Verification items for the finished model (mm, model axes). Face numbers are marked on the shaded views. A direction names the side the tool comes from. Round coordinates to 2 decimals unless told otherwise and drop trailing zeros. Write each loop counter-clockwise with the first axis right and the second up, starting at its lowest first coordinate (ties: lowest second). Pieces come first, ordered by that corner, then holes. Notation, with made-up numbers: M 65,79 L 73,79 A27 cw 73,104 Z; hole C -30,2 d5. An arc over 180 degrees is marked long. One line per question, with ' | ' between items. Start each with the question number.
Q1. Cross-section at B-B (y = 52). Record the boundary of the cut face in (x, z).
Q2. Thickness scan on line 1 along Z through (x, y) = (25, -78); line 2 along Y through (x, z) = (-16, 42.5); line 3 along Z through (x, y) = (33, 147). Record the ranges inside material, lowest first. Write a range as from..to.
Q3. Tool access check on the marked faces 1, 2 and 3. Record the directions out of +Z, -Z, +X, -X, +Y, -Y that give a thin tool (end or side, any length) a straight path to the whole face; none if there is none.
Q4. Gauge pin test, flat ends, axial feed: pin 1 (2 mm diameter, centred on x = 14, z = -43.5, fed in from +Y); pin 2 (3 mm diameter, centred on y = -14, z = 30, fed in from -X); pin 3 (6 mm diameter, centred on x = 25, z = 0, fed in from -Y); pin 4 (16.5 mm diameter, centred on x = 25, z = 0, fed in from +Y). Record the tip position at first contact, or that the pin passes through.
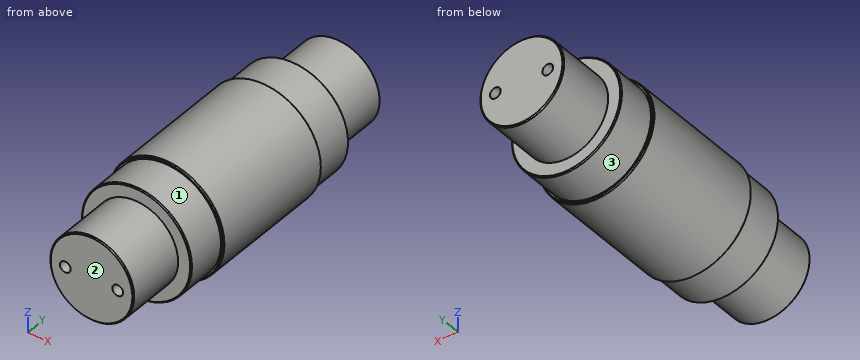
from build123d import *

# Parameters (mm, degrees)
F0_R      = 55
F1_DEPTH  = 125
F2_R      = 52.5
F3_DEPTH  = 38
F4_R      = 40
F5_DEPTH  = 57
F6_R      = 52.5
F7_DEPTH  = 38
F8_R      = 40
F9_DEPTH  = 57
F10_SIZE  = 1
F11_SIZE  = 1
F12_SIZE  = 1
F13_SIZE  = 1
F14_SIZE  = 1
F15_SIZE  = 1
F17_D     = 10.3
F17_DEPTH = 30.25
F17_TIP   = 3.094432188
F19_D     = 10.3
F19_DEPTH = 17.25
F19_TIP   = 3.094432188


with BuildPart() as f1:
    # F0 (on Front) → F1 (new body)
    with BuildSketch(Plane.XZ):
        Circle(F0_R)
    extrude(amount=-F1_DEPTH)

    # F2 (on face) → F3 (join)
    with BuildSketch(Plane.XZ):
        Circle(F2_R)
    extrude(amount=F3_DEPTH)

    # F4 (on face) → F5 (join)
    with BuildSketch(Plane.XZ.offset(38)):
        Circle(F4_R)
    extrude(amount=F5_DEPTH)

    # F6 (on face) → F7 (join)
    with BuildSketch(Plane(origin=(0, 125, 0), x_dir=(-1, 0, 0), z_dir=(0, 1, 0))):
        Circle(F6_R)
    extrude(amount=F7_DEPTH)

    # F8 (on face) → F9 (join)
    with BuildSketch(Plane(origin=(0, 163, 0), x_dir=(-1, 0, 0), z_dir=(0, 1, 0))):
        Circle(F8_R)
    extrude(amount=F9_DEPTH)

    # F10
    f10_edges = [f1.edges().sort_by_distance(p)[0] for p in [
        (-40, -95, 0),
    ]]
    chamfer(f10_edges, length=F10_SIZE)

    # F11
    f11_edges = [f1.edges().sort_by_distance(p)[0] for p in [
        (-52.5, -38, 0),
    ]]
    chamfer(f11_edges, length=F11_SIZE)

    # F12
    f12_edges = [f1.edges().sort_by_distance(p)[0] for p in [
        (-55, 0, 0),
    ]]
    chamfer(f12_edges, length=F12_SIZE)

    # F13
    f13_edges = [f1.edges().sort_by_distance(p)[0] for p in [
        (40, 220, 0),
    ]]
    chamfer(f13_edges, length=F13_SIZE)

    # F14
    f14_edges = [f1.edges().sort_by_distance(p)[0] for p in [
        (52.5, 163, 0),
    ]]
    chamfer(f14_edges, length=F14_SIZE)

    # F15
    f15_edges = [f1.edges().sort_by_distance(p)[0] for p in [
        (-55, 125, 0),
    ]]
    chamfer(f15_edges, length=F15_SIZE)

    # F17
    with Locations(Plane.XZ.offset(95)):
        with Locations((-25, 0), (25, 0)):
            Hole(F17_D / 2, depth=F17_DEPTH)
            with Locations((0, 0, -(F17_DEPTH + F17_TIP / 2))):  # 118° drill point
                Cone(0, F17_D / 2, F17_TIP, mode=Mode.SUBTRACT)

    # F19
    with Locations(Plane(origin=(0, 220, 0), x_dir=(-1, 0, 0), z_dir=(0, 1, 0))):
        with Locations((-25, 0), (25, 0)):
            Hole(F19_D / 2, depth=F19_DEPTH)
            with Locations((0, 0, -(F19_DEPTH + F19_TIP / 2))):  # 118° drill point
                Cone(0, F19_D / 2, F19_TIP, mode=Mode.SUBTRACT)


solid = f1.part
Determined:
1) outline: C 0,0 d110
2) line 1: z = -31.22..-5.15, 5.15..31.22 | line 2: y = -38..163 | line 3: z = -40.83..40.83
3) face 1: -Y | face 2: +Z, -Z, +X, -X, -Y | face 3: +Y
4) pin 1: stops at y = 163 | pin 2: stops at x = -44.09 | pin 3: stops at y = -63.46 | pin 4: stops at y = 220
